Could you check a few things on this model? Use its own coordinates, in mm. Face numbers are marked on the shaded views. A direction names the side the tool comes from. Round coordinates to 2 decimals unless told otherwise and drop trailing zeros. Loops run counter-clockwise (first coordinate to the right, second up) from the corner with the lowest first, then second, coordinate; pieces in that order, holes last. Notation, with made-up numbers: (70, -22) -> (129, -22) arc R15 cw to (129, -14) -> close; hole circle Ø8 at (-15, -38.5). An arc over 180 degrees is marked (long way). One line per item, written item: value.
```python
from build123d import *

# Parameters (mm, degrees)
CROQUIS1_W                  = 48
CROQUIS1_H                  = 30
SALIENTE_EXTRUIR1_DEPTH     = 14
CORTAR_EXTRUIR1_DEPTH       = 37
REDONDEO2_R                 = 7
CROQUIS3_W                  = 20
CROQUIS3_H                  = 16
CORTAR_EXTRUIR2_DEPTH       = 3
CROQUIS5_R                  = 1.5
CORTAR_EXTRUIR3_DEPTH       = 12
CROQUIS10_R                 = 6.927737764
CORTAR_EXTRUIR9_DEPTH       = 3
CORTAR_EXTRUIR10_REACH      = 54.494
CORTAR_EXTRUIR10_END_RADIUS = 6.927737764
CROQUIS11_R                 = 3
SALIENTE_EXTRUIR5_DEPTH     = 4
CORTAR_EXTRUIR14_REACH      = 59.227
CROQUIS12_R                 = 3.5
CORTAR_EXTRUIR16_DEPTH      = 22
CROQUIS16_R                 = 2
CORTAR_EXTRUIR17_DEPTH      = 2
CROQUIS17_W                 = 3
CROQUIS17_H                 = 5
CORTAR_EXTRUIR18_DEPTH      = 3
CROQUIS18_R                 = 1.7
CORTAR_EXTRUIR19_DEPTH      = 4
REDONDEO3_R                 = 10


with BuildPart() as part:
    # Croquis1 → Saliente-Extruir1 (new body)
    with BuildSketch(Plane.XY):
        with Locations((-19.976765257, 0.987352556)):
            Rectangle(CROQUIS1_W, CROQUIS1_H)
    extrude(amount=SALIENTE_EXTRUIR1_DEPTH)

    # Croquis2 → Cortar-Extruir1 (cut)
    with BuildSketch(Plane(origin=(4.023234743, 0, 0), x_dir=(0, 0, -1), z_dir=(1, 0, 0))):
        with BuildLine():
            ThreePointArc((-14, -10.012647444), (-9.618950039, 0.987352556), (-14, 11.987352556))
            Line((-14, 11.987352556), (-14, -10.012647444))
        make_face()
    extrude(amount=-CORTAR_EXTRUIR1_DEPTH, mode=Mode.SUBTRACT)

    # Redondeo2
    # the kernel refuses this fillet: 7 mm, written as the material it takes off along each edge
    with BuildSketch(Plane(origin=(-2.976765257, -7.012647444, 7), x_dir=(0, 0, -1), z_dir=(1, 0, 0))) as redondeo2_piece_1_section:
        Polygon((0, 0), (REDONDEO2_R, 0), (REDONDEO2_R, -REDONDEO2_R), (0, -REDONDEO2_R), align=None)
    redondeo2_piece_1 = extrude(amount=REDONDEO2_R, mode=Mode.PRIVATE)
    redondeo2_piece_1 = redondeo2_piece_1 - Plane(origin=(-2.976765257, -7.012647444, 7), x_dir=(0, 0.7071067811865475, 0.7071067811865475), z_dir=(1, 0, 0)) * Sphere(REDONDEO2_R, mode=Mode.PRIVATE)
    add(redondeo2_piece_1, mode=Mode.SUBTRACT)
    with BuildSketch(Plane(origin=(-2.976765257, 8.987352556, 7), x_dir=(1, 0, 0), z_dir=(0, 1, 0))) as redondeo2_piece_2_section:
        Polygon((0, 0), (REDONDEO2_R, 0), (REDONDEO2_R, REDONDEO2_R), (0, REDONDEO2_R), align=None)
    redondeo2_piece_2 = extrude(amount=REDONDEO2_R, mode=Mode.PRIVATE)
    redondeo2_piece_2 = redondeo2_piece_2 - Plane(origin=(-2.976765257, 8.987352556, 7), x_dir=(-0.7071067811865475, 0, 0.7071067811865475), z_dir=(0, 1, 0)) * Sphere(REDONDEO2_R, mode=Mode.PRIVATE)
    add(redondeo2_piece_2, mode=Mode.SUBTRACT)
    with BuildSketch(Plane(origin=(-2.976765257, -14.012647444, 0), x_dir=(0, 1, 0), z_dir=(-1, 0, 0))) as redondeo2_piece_3:
        with BuildLine():
            CenterArc((REDONDEO2_R, -REDONDEO2_R), REDONDEO2_R, 90, 90)
            Line((0, -REDONDEO2_R), (0, 0))
            Line((0, 0), (REDONDEO2_R, 0))
        make_face()
    extrude(amount=58.5, mode=Mode.SUBTRACT)
    with BuildSketch(Plane(origin=(4.023234743, 8.987352556, 0), x_dir=(0, 0, 1), z_dir=(0, -1, 0))) as redondeo2_piece_4:
        with BuildLine():
            CenterArc((REDONDEO2_R, REDONDEO2_R), REDONDEO2_R, 180, 90)
            Line((0, REDONDEO2_R), (0, 0))
            Line((0, 0), (REDONDEO2_R, 0))
        make_face()
    extrude(amount=16, mode=Mode.SUBTRACT)
    with BuildSketch(Plane(origin=(-61.476765257, 15.987352556, 0), x_dir=(0, 0, 1), z_dir=(1, 0, 0))) as redondeo2_piece_5:
        with BuildLine():
            CenterArc((REDONDEO2_R, REDONDEO2_R), REDONDEO2_R, 180, 90)
            Line((0, REDONDEO2_R), (0, 0))
            Line((0, 0), (REDONDEO2_R, 0))
        make_face()
    extrude(amount=58.5, mode=Mode.SUBTRACT)
    with BuildSketch(Plane(origin=(4.023234743, 15.987352556, 7), x_dir=(-1, 0, 0), z_dir=(0, 0, 1)), Plane(origin=(4.023234743, -14.012647444, 7), x_dir=(0, 1, 0), z_dir=(0, 0, 1))) as redondeo2_piece_6:
        with BuildLine():
            CenterArc((REDONDEO2_R, REDONDEO2_R), REDONDEO2_R, 180, 90)
            Line((0, REDONDEO2_R), (0, 0))
            Line((0, 0), (REDONDEO2_R, 0))
        make_face()
    extrude(amount=24.5, mode=Mode.SUBTRACT)

    # Croquis3 → Cortar-Extruir2 (cut)
    with BuildSketch(Plane(origin=(0, 0, 0), x_dir=(-1, 0, 0), z_dir=(0, 0, -1))):
        with Locations((18.976765257, 0.987352556)):
            Rectangle(CROQUIS3_W, CROQUIS3_H)
    extrude(amount=-CORTAR_EXTRUIR2_DEPTH, mode=Mode.SUBTRACT)

    # Croquis5 → Cortar-Extruir3 (cut)
    with BuildSketch(Plane(origin=(0, 0, 0), x_dir=(-1, 0, 0), z_dir=(0, 0, -1))):
        with Locations((20.076765257, 0.987352556)):
            Circle(CROQUIS5_R)
        with Locations((15.876765257, 0.987352556)):
            Circle(CROQUIS5_R)
    extrude(amount=-CORTAR_EXTRUIR3_DEPTH, mode=Mode.SUBTRACT)

    # Croquis10 → Cortar-Extruir9 (cut)
    with BuildSketch(Plane(origin=(0, 0, 3), x_dir=(-1, 0, 0), z_dir=(0, 0, -1))):
        with Locations((17.983902927, 0.987352556)):
            Circle(CROQUIS10_R)
    extrude(amount=-CORTAR_EXTRUIR9_DEPTH, mode=Mode.SUBTRACT)

    # Cortar-Extruir10: up to this cylinder (the profile starts outside it)
    cortar_extruir10_end = Plane(origin=(-17.983902927, 0.987352556, 4.236484), z_dir=(0, 0, -1)) * Cylinder(CORTAR_EXTRUIR10_END_RADIUS, 123.843475528, mode=Mode.PRIVATE)
    # Croquis11 → Cortar-Extruir10 (cut, up to the surface)
    with BuildSketch(Plane.ZY.offset(43.976765257), mode=Mode.PRIVATE) as cortar_extruir10_sk1:
        with Locations(Location((4.236484056, 0.987352556, 0), (0, 0, 270))):
            Circle(CROQUIS11_R)
    cortar_extruir10_tool1 = extrude(cortar_extruir10_sk1.sketch, amount=-CORTAR_EXTRUIR10_REACH, mode=Mode.PRIVATE) - cortar_extruir10_end
    add(cortar_extruir10_tool1.solids().sort_by_distance((-43.976765, 0.987353, 4.236484))[0], mode=Mode.SUBTRACT)

    # Croquis14 → Saliente-Extruir5 (add)
    with BuildSketch(Plane.XZ.offset(14.012647444)):
        with BuildLine():
            ThreePointArc((-33.976765257, 16), (-38.976765257, 21), (-43.976765257, 16))
            ThreePointArc((-43.976765257, 16), (-43.871296822, 14.978451782), (-43.559340952, 14))
            Line((-43.559340952, 14), (-34.394189562, 14))
            ThreePointArc((-34.394189562, 14), (-34.082233692, 14.978451782), (-33.976765257, 16))
        make_face()
        with BuildLine():
            Line((-34.394189562, 14), (-43.559340952, 14))
            ThreePointArc((-43.559340952, 14), (-38.976765257, 11), (-34.394189562, 14))
        make_face()
        with BuildLine():
            ThreePointArc((-43.559340952, 14), (-43.871296822, 14.978451782), (-43.976765257, 16))
            Line((-43.976765257, 16), (-43.976765257, 14))
            Line((-43.976765257, 14), (-43.559340952, 14))
        make_face()
    saliente_extruir5 = extrude(amount=-SALIENTE_EXTRUIR5_DEPTH)

    # Simetría1: Saliente-Extruir5 across plane
    add(saliente_extruir5.mirror(Plane.ZX.offset(0.987352556)))

    # Cortar-Extruir14: up to this face of the body (flat: up to its plane)
    cortar_extruir14_end = Plane(part.part.faces().sort_by_distance((-38.999365489, 11.987352556, 17.080483699))[0])
    # Croquis12 → Cortar-Extruir14 (cut, up to the picked face)
    with BuildSketch(Plane.XZ.offset(14.012647444), mode=Mode.PRIVATE) as cortar_extruir14_sk1:
        with Locations(Location((-38.976765257, 16, 0), (0, 0, 270))):
            Circle(CROQUIS12_R)
    cortar_extruir14_tool1 = split(extrude(cortar_extruir14_sk1.sketch, amount=-CORTAR_EXTRUIR14_REACH, mode=Mode.PRIVATE), bisect_by=cortar_extruir14_end, keep=Keep.BOTH, mode=Mode.PRIVATE)
    add(cortar_extruir14_tool1.solids().sort_by(Axis((-38.976765, -14.012647, 16), (0, 1, 0)))[0], mode=Mode.SUBTRACT)

    # Croquis15 → Cortar-Extruir16 (cut)
    with BuildSketch(Plane.XZ.offset(10.012647444)):
        Polygon((-43.976765257, 16), (-43.976765257, 12), (-41.976765257, 16), align=None)
    extrude(amount=-CORTAR_EXTRUIR16_DEPTH, mode=Mode.SUBTRACT)

    # Croquis16 → Cortar-Extruir17 (cut)
    with BuildSketch(Plane(origin=(0, 0, 6), x_dir=(-1, 0, 0), z_dir=(0, 0, -1))):
        with Locations((15.876765257, 0.987352556)):
            Circle(CROQUIS16_R)
        with Locations((20.076765257, 0.987352556)):
            Circle(CROQUIS16_R)
    extrude(amount=-CORTAR_EXTRUIR17_DEPTH, mode=Mode.SUBTRACT)

    # Croquis17 → Cortar-Extruir18 (cut)
    with BuildSketch(Plane(origin=(0, 0, 0), x_dir=(-1, 0, 0), z_dir=(0, 0, -1))):
        with Locations((30.476765257, 0.987352556)):
            Rectangle(CROQUIS17_W, CROQUIS17_H)
    extrude(amount=-CORTAR_EXTRUIR18_DEPTH, mode=Mode.SUBTRACT)

    # Croquis18 → Cortar-Extruir19 (cut)
    with BuildSketch(Plane(origin=(0, 15.987352556, 0), x_dir=(1, 0, 0), z_dir=(0, 1, 0))):
        with Locations(Location((-38.976765257, -16, 0), (0, 0, 270))):
            Circle(CROQUIS18_R)
    extrude(amount=-CORTAR_EXTRUIR19_DEPTH, mode=Mode.SUBTRACT)

    # Redondeo3
    # the kernel refuses this fillet: 10 mm, written as the material it adds along each edge
    with BuildSketch(Plane(origin=(-32.976765257, 0.987352556, 25.618950039), x_dir=(0, -0.7314644805706508, 0.6818795448343558), z_dir=(0, 0.6818795448343558, 0.7314644805706508))) as redondeo3_piece_1_section:
        with BuildLine():
            CenterArc((16 - REDONDEO3_R, REDONDEO3_R), REDONDEO3_R, 270, 90)
            Line((16 - REDONDEO3_R, 0), (16, 0))
            Line((16, 0), (16, REDONDEO3_R))
        make_face()
    redondeo3_piece_1 = revolve(axis=Axis((-32.976765257, 0.987352556, 25.618950039), (1, 0, 0)), revolution_arc=265.981384943, mode=Mode.PRIVATE)
    redondeo3_piece_1 = split(redondeo3_piece_1, bisect_by=Plane(origin=(-29.991953526, 0.987352592, 14), z_dir=(0, 0, -1)), keep=Keep.TOP, mode=Mode.PRIVATE)
    add(redondeo3_piece_1)


solid = part.part
```
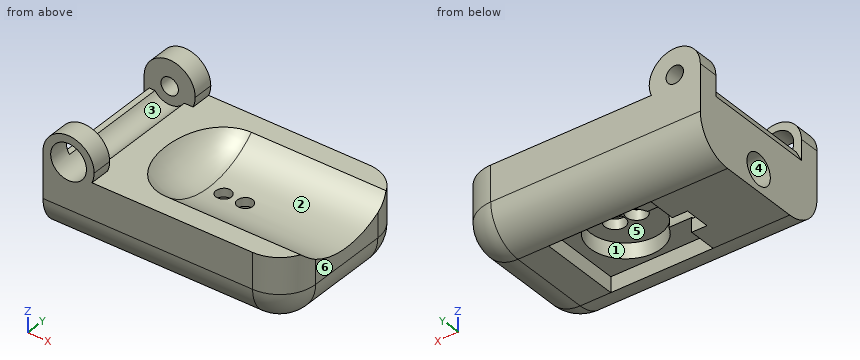
Item 1: If we section it at B-B on x = -15: List the corners of the cut face in (y, z) for me, plus the area to 3 significant figures.
Output:
outline: (-14.01, 7) arc R7 ccw to (-7.01, 0) -> (-7.01, 3) -> (-5.26, 3) -> (-5.26, 6) -> (-0.81, 6) -> (-0.81, 8) -> (-0.23, 8) -> (-0.23, 9.67) arc R16 cw to (-10.01, 14) -> (-14.01, 14) -> close; (2.2, 8) -> (2.78, 8) -> (2.78, 6) -> (7.24, 6) -> (7.24, 3) -> (8.99, 3) -> (8.99, 0) arc R7 ccw to (15.99, 7) -> (15.99, 14) -> (11.99, 14) arc R16 cw to (2.2, 9.67) -> close
area: 236 mm²
Item 2: If we section it at A-A on x = -3.5: List the corners of the cut face in (y, z) for me, plus the area to 3 significant figures.
Output:
outline: (-14.01, 7) arc R7 ccw to (-7.01, 0) -> (8.99, 0) arc R7 ccw to (15.99, 7) -> (15.99, 14) -> (11.99, 14) arc R16 cw to (-10.01, 14) -> (-14.01, 14) -> close
area: 333 mm²
Item 3: Will these pins go through, and if not, where does the flat tip stop? pin 1 Ø5 at (x, y) = (-15.5, -2) entering from -Z; pin 2 Ø0.8 at (x, z) = (-31, 2) entering from -Y; pin 3 Ø1.5 at (x, y) = (-27.5, 11.5) entering from -Z.
Output:
pin 1: stops at z = 6
pin 2: stops at y = -12.29
pin 3: stops at z = 0.23
Item 4: If we section it at D-D on x = -10: List the corners of the cut face in (y, z) for me.
Output:
outline: (-14.01, 7) arc R7 ccw to (-7.01, 0) -> (-7.01, 3) -> (8.99, 3) -> (8.99, 0) arc R7 ccw to (15.99, 7) -> (15.99, 14) -> (11.99, 14) arc R16 cw to (-10.01, 14) -> (-14.01, 14) -> close
Item 5: If we mould it in two halves opening along Z, with no side actions, what happens to the marked faces 4, 5 and 6? For each: released by +Z, released by -Z, zero draft, split by the parting line, or undercut.
Output:
face 4: undercut
face 5: released by -Z
face 6: zero draft
Item 6: For the marked faces 1, 2 and 3, which set-ups out of +Z, -Z, +X, -X, +Y, -Y let a thin tool reach every point of the face, with its end or its side?
Output:
face 1: -Z
face 2: +Z, +X
face 3: -Y
Item 7: I need wall thicknesses on line 1 (Y direction, x = -34.5, z = 14.5); line 2 (X direction, y = -11, z = 16); line 3 (Y direction, x = -18, z = 11.5). Which ranges of each line are inside material? Lowest first, please. Write a range as from..to.
Output:
line 1: y = -14.01..-10.01, 11.99..15.99
line 2: x = -43.98..-42.48, -35.48..-33.98
line 3: y = -14.01..-6.54, 8.51..15.99
Item 8: If we section it at C-C on z = 1.75: List the corners of the cut face in (x, y) for me, plus the area to 3 significant figures.
Output:
outline: (-43.98, -11.64) -> (-2.98, -11.64) arc R4.63 ccw to (1.65, -7.01) -> (1.65, 8.99) arc R4.63 ccw to (-2.98, 13.62) -> (-43.98, 13.62) -> (-43.98, 2.67) -> (-31.98, 2.67) -> (-31.98, 3.49) -> (-28.98, 3.49) -> (-28.98, 8.99) -> (-8.98, 8.99) -> (-8.98, -7.01) -> (-28.98, -7.01) -> (-28.98, -1.51) -> (-31.98, -1.51) -> (-31.98, -0.69) -> (-43.98, -0.69) -> close
area: 768 mm²
